from build123d import *

# Parameters (mm, degrees)
SKETCH11_W               = 9.398
SKETCH11_H               = 9.398
STRUCTURAL_MEMBER1_DEPTH = 260.096


with BuildPart() as part:
    # Sketch11 → Structural Member1 (new body)
    with BuildSketch(Plane.YZ):
        with BuildLine():
            Line((-5.55625, 6.35), (5.55625, 6.35))
            ThreePointArc((5.55625, 6.35), (6.117516008, 6.117516008), (6.35, 5.55625))
            Line((6.35, 5.55625), (6.35, -5.55625))
            ThreePointArc((6.35, -5.55625), (6.117516008, -6.117516008), (5.55625, -6.35))
            Line((5.55625, -6.35), (-5.55625, -6.35))
            ThreePointArc((-5.55625, -6.35), (-6.117516008, -6.117516008), (-6.35, -5.55625))
            Line((-6.35, -5.55625), (-6.35, 5.55625))
            ThreePointArc((-6.35, 5.55625), (-6.117516008, 6.117516008), (-5.55625, 6.35))
        make_face()
        Rectangle(SKETCH11_W, SKETCH11_H, mode=Mode.SUBTRACT)
    extrude(amount=STRUCTURAL_MEMBER1_DEPTH)


solid = part.part
Check sheet for the modelled part. Datum: model origin and axes. Units: mm. A direction names the side the tool comes from. Round coordinates to 2 decimals unless told otherwise and drop trailing zeros. Write each loop counter-clockwise with the first axis right and the second up, starting at its lowest first coordinate (ties: lowest second). Pieces come first, ordered by that corner, then holes. Notation, with made-up numbers: (89, 35) - (121, 35) arc R16 ccw to (121, 41) - close; hole circle Ø4 at (62.25, 56.25). An arc over 180 degrees is marked (long way). Return JSON: item names as keys, results as strings.
Q1. Cross-section at B-B (x = 114). Record the boundary of the cut face in (y, z), then the cut area to 3 significant figures.
Returned:
{"outline": "(-6.35, -5.56) arc R0.79 ccw to (-5.56, -6.35) - (5.56, -6.35) arc R0.79 ccw to (6.35, -5.56) - (6.35, 5.56) arc R0.79 ccw to (5.56, 6.35) - (-5.56, 6.35) arc R0.79 ccw to (-6.35, 5.56) - close; hole (-4.7, -4.7) - (4.7, -4.7) - (4.7, 4.7) - (-4.7, 4.7) - close", "area": "72.4 mm²"}
Q2. Access from +Z, -Z, +X, -X, +Y, -Y to the whole of each face (thin tool, end or side, straight path). Record for faces 1 (the flat face through (128, 0, -6.35)), 2 (the flat face through (128, 0, 4.699)).
Returned:
{"face 1": "-Z, +X, -X, +Y, -Y", "face 2": "+X, -X"}
Q3. Draft check along Z on faces 3 (the flat face through (128, 0, 6.35)), 4 (the flat face through (128, 0, -4.699)), 5 (the flat face through (260.096, -6, 0)). Enter one of: released by +Z, released by -Z, zero draft, split by the parting line, or undercut.
Returned:
{"face 3": "released by +Z", "face 4": "undercut", "face 5": "zero draft"}
Q4. Scan line: L1, parallel to Y at x = 155.5, z = 4. Record every from-to range of solid material in increasing order. Write a range as from..to.
Returned:
{"L1": "y = -6.35..-4.7, 4.7..6.35"}
Q5. Cross-section at A-A (y = -2). Record the boundary of the cut face in (x, z), then the cut area to 3 significant figures.
Returned:
{"outline": "(0, -6.35) - (260.1, -6.35) - (260.1, -4.7) - (0, -4.7) - close; (0, 4.7) - (260.1, 4.7) - (260.1, 6.35) - (0, 6.35) - close", "area": "859 mm²"}
